CAD build for the part. Positions are in the model's coordinates, mm. Face numbers are marked on the shaded views. A direction names the side the tool comes from. Coordinates: 2 decimals unless noted, no trailing zeros. Loops run counter-clockwise (first coordinate to the right, second up) from the corner with the lowest first, then second, coordinate; pieces in that order, holes last. Notation, with made-up numbers: (5.5, -21) - (21.5, -21) arc R27 ccw to (21.5, 5) - close; hole circle Ø9 at (49, 49.5). An arc over 180 degrees is marked (long way). Put each result on its own line as item: value.
Autodesk Inventor part; units mm, degrees
ref_plane "YZ Plane" through (0, 0, 0) normal (1, 0, 0) x (0, 1, 0)
ref_plane "XZ Plane" through (0, 0, 0) normal (0, 1, 0) x (-1, 0, 0)
ref_plane "XY Plane" through (0, 0, 0) normal (0, 0, 1) x (1, 0, 0)
sketch "Sketch1" plane through (0, 0, 0) normal (0, 0, 1) x (1, 0, 0)
  circle A0 centre (0, 0) radius 28.575
  dimension "d0" = 57.15
extrude "Extrusion1" add sketch "Sketch1" along normal blind 57.15
sketch "Sketch2" plane through (0, 0, 0) normal (0, 0, -1) x (-1, 0, 0)
  circle A0 centre (0, 0) radius 28.575
  line L0 (-25.4, 25.4) -> (25.4, 25.4)
  line L1 (25.4, 25.4) -> (25.4, -25.4)
  line L2 (25.4, -25.4) -> (-25.4, -25.4)
  line L3 (-25.4, -25.4) -> (-25.4, 25.4)
  dimension "d4" = 25.4
  dimension "d5" = 25.4
  dimension "d6" = 25.4
  dimension "d7" = 25.4
extrude "Extrusion2" add sketch "Sketch2" along normal blind 88.9 contours L1 A0 L2 L3 L0 | A0 L0 L1 | L1 L2 A0 | A0 L3 L0 | L2 L3 A0
sketch "Sketch3" plane through (0, 0, -88.9) normal (0, 0, -1) x (-1, 0, 0)
  circle A0 centre (0, 0) radius 28.575
  dimension "d10" = 57.15
extrude "Extrusion3" add sketch "Sketch3" along normal blind 3.175
sketch "Sketch4" plane through (0, 0, -92.075) normal (0, 0, -1) x (-1, 0, 0)
  circle A0 centre (0, 0) radius 12.7
  dimension "d13" = 25.4
extrude "Extrusion4" add sketch "Sketch4" along normal blind 25.4
sketch "Sketch5" plane through (0, 0, -117.475) normal (0, 0, -1) x (-1, 0, 0)
  circle A0 centre (0, 0) radius 28.575
  dimension "d16" = 57.15
extrude "Extrusion5" add sketch "Sketch5" along normal blind 3.175
fillet "Fillet1" radius 9.525 4 edges at (25.4, 25.4, -44.45) (-25.4, 25.4, -44.45) (25.4, -25.4, -44.45) (-25.4, -25.4, -44.45)
properties part number "ScissorLiftMotorApproximation"
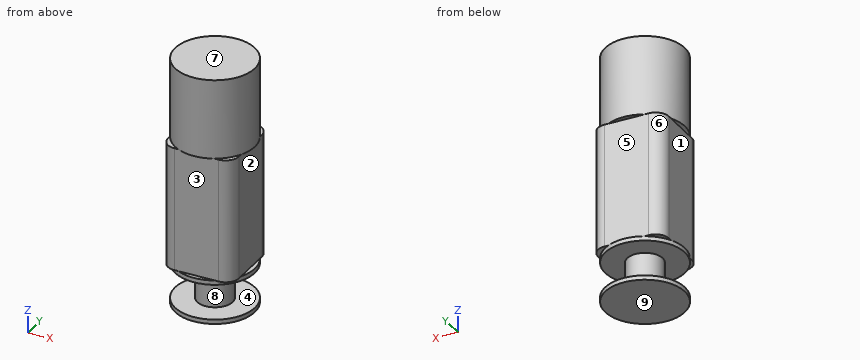
Q1. Slice it at D-D, the plane z = -77.5. Give the cut face in (x, y) (3 decimals), then the cut area to 3 significant figures.
Determined:
outline: (-25.4, -15.875) arc R9.525 ccw to (-15.875, -25.4) - (15.875, -25.4) arc R9.525 ccw to (25.4, -15.875) - (25.4, 15.875) arc R9.525 ccw to (15.875, 25.4) - (-15.875, 25.4) arc R9.525 ccw to (-25.4, 15.875) - close
area: 2,500 mm2
Q2. Pin check, flat tips, straight feed: pin 1 Ø12 at (x, z) = (-2.5, -7.5) entering from -Y; pin 2 Ø5 at (y, z) = (-22, -31) entering from +X; pin 3 Ø6 at (x, z) = (-5.5, -25.5) entering from +Y. Stop position of each tip, or through.
Determined:
pin 1: y = -25.4
pin 2: x = 24.68
pin 3: y = 25.4
Q3. Tool access for the marked faces 1, 2, 3, 4 and 5: list every direction of +Z, -Z, +X, -X, +Y, -Y with a clear straight run to the whole face (end or side of a thin tool).
Determined:
face 1: -X, +Y, -Y
face 2: +X, +Y, -Y
face 3: +X, -X, -Y
face 4: none
face 5: +X, -X, +Y
Q4. Mould opens along Z. For the marked faces 6, 7, 8 and 9 say: +Z half, -Z half, draft (parallel to the pull), parting line (faces both ways), or undercut.
Determined:
face 6: draft
face 7: +Z half
face 8: undercut
face 9: -Z half
Q5. Wall check: L1, parallel to Z at x = -11, y = 13 (3 decimals); L2, parallel to Y at x = 3, z = -52. Give the ranges that are in metal, low to high. Write a range as from..to.
Determined:
L1: -120.65..-117.475, -92.075..57.15
L2: -25.4..25.4
Q6. Slice it at B-B, the plane y = -19. Give the cut face in (x, z) (3 decimals).
Determined:
outline: (-24.873, -88.9) - (-21.343, -88.9) - (-21.343, -92.075) - (21.343, -92.075) - (21.343, -88.9) - (24.873, -88.9) - (24.873, 0) - (21.343, 0) - (21.343, 57.15) - (-21.343, 57.15) - (-21.343, 0) - (-24.873, 0) - close; (-21.343, -120.65) - (21.343, -120.65) - (21.343, -117.475) - (-21.343, -117.475) - close
Q7. Slice it at A-A, the plane x = 0. Give the cut face in (y, z) (3 decimals), then the cut area to 3 significant figures.
Determined:
outline: (-28.575, -120.65) - (28.575, -120.65) - (28.575, -117.475) - (12.7, -117.475) - (12.7, -92.075) - (28.575, -92.075) - (28.575, -88.9) - (25.4, -88.9) - (25.4, 0) - (28.575, 0) - (28.575, 57.15) - (-28.575, 57.15) - (-28.575, 0) - (-25.4, 0) - (-25.4, -88.9) - (-28.575, -88.9) - (-28.575, -92.075) - (-12.7, -92.075) - (-12.7, -117.475) - (-28.575, -117.475) - close
area: 8,790 mm2
